Part model, mm, in its own coordinate system. Coordinates: 2 decimals unless noted, no trailing zeros. Loops run counter-clockwise (first coordinate to the right, second up) from the corner with the lowest first, then second, coordinate; pieces in that order, holes last. Notation, with made-up numbers: M 46,51.5 L 81,51.5 A13 cw 81,58.5 Z; hole C 37.25,2.5 d3. An arc over 180 degrees is marked long. Answer as a JSON object with one key per item and string values. Group by question number.
1. Saw through at A-A on z = 66. Write the cut outline in (x, y).
2. Drill centre lines: L1, parallel to X at y = 1.25, z = 54; L2, parallel to X at y = 4.75, z = 79.5; L3, parallel to Z at x = 321.5, y = 0.5. Where is each one in solid material? Low to high.
3. Drop a flat-ended pin along its axis: pin 1 Ø1 at (y, z) = (4.5, 64) entering from -X. Give the stop position or say it passes through.
4. Saw through at B-B on y = 3.75. Write the cut outline in (x, z), then the cut area to 3 significant figures.
from build123d import *

# Parameters (mm, degrees)
BOSS_EXTRUDE1_DEPTH = 6.35
CUT_EXTRUDE1_DEPTH  = 609.6


with BuildPart() as part:
    # Sketch1 → Boss-Extrude1 (new body)
    with BuildSketch(Plane(origin=(0, 0, 0), x_dir=(1, 0, 0), z_dir=(0, 1, 0))):
        Polygon((-381, -88.9), (-469.9, 0), (469.9, 0), (381, -88.9), align=None)
    extrude(amount=BOSS_EXTRUDE1_DEPTH)

    # Sketch2 → Cut-Extrude1 (cut)
    with BuildSketch(Plane(origin=(0, 6.35, 0), x_dir=(1, 0, 0), z_dir=(0, 1, 0))):
        Polygon((-380.097438789, 0), (-291.197438789, -88.9), (-381, -88.9), (-469.9, 0), align=None)
    cut_extrude1 = extrude(amount=-CUT_EXTRUDE1_DEPTH, mode=Mode.SUBTRACT)

    # Mirror1: Cut-Extrude1 across plane
    add(cut_extrude1.mirror(Plane(origin=(0, 0, 0), x_dir=(0, 0, 1), z_dir=(1, 0, 0))), mode=Mode.SUBTRACT)


solid = part.part
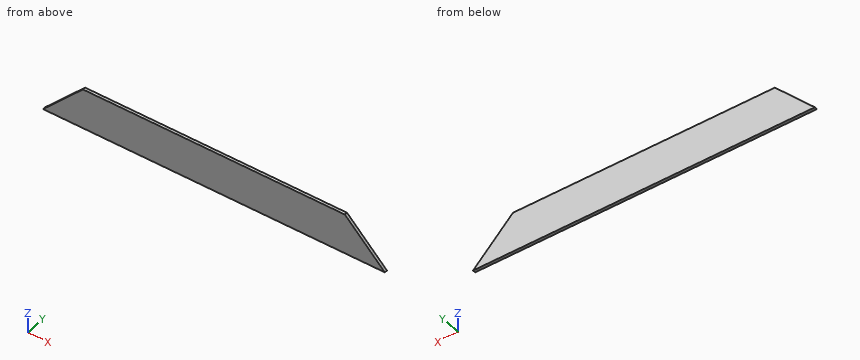
Outcome:
{
 "1": {"outline": "M -314.1,0 L 314.1,0 L 314.1,6.35 L -314.1,6.35 Z"},
 "2": {"L1": "x = -326.1 to 326.1", "L2": "x = -300.6 to 300.6", "L3": "z = 0 to 58.6"},
 "3": {"pin 1": "stops at x = -316.6"},
 "4": {"outline": "M -380.1,0 L 380.1,0 L 291.2,88.9 L -291.2,88.9 Z", "area": "59,700 mm²"}
}
